Design review of the part shown in the three views and the two pictorial views. Dimensions are in mm from the part's minimum x, y and z. Give positions to 0.01 mm unless a question says otherwise; leave off trailing zeros. Loops run counter-clockwise (first coordinate to the right, second up) from the corner with the lowest first, then second, coordinate; pieces in that order, holes last. Notation, with made-up numbers: (-29.5, -16) -> (24.5, -16) arc R32 ccw to (24.5, 10) -> close; hole circle Ø2 at (85.25, 41.5). An arc over 180 degrees is marked (long way). Use CSV: the item, a comma, the result in double quotes. Start each with the question number.
Item 1: Wall thickness on line 1 along Y through (x, z) = (20.5, 67); line 2 along X through (y, z) = (14.25, 53); line 3 along X through (y, z) = (1, 57.5): over which ranges is each line inside the solid? List them lowest first. Write a range as from..to.
Item 2: The part is to be moulded in two halves that separate along Y. For the marked faces 1, 2, 3 and 4, say which applies: +Y half, -Y half, draft (parallel to the pull), parting line (faces both ways), or undercut.
Item 3: We need section D-D (y = 3). State the section outline as (x, z) points.
Item 4: We need section B-B (y = 9.5). State the section outline as (x, z) points, plus the area to 3 significant figures.
Item 5: We need section A-A (z = 6). State the section outline as (x, y) points.
Item 6: Clearance check with flat-ended pins moving along their axes: pin 1 (12 mm diameter, centred on y = 6, z = 50, fed in from +X); pin 2 (3 mm diameter, centred on x = 48, y = 8, fed in from +Z); pin 3 (8 mm diameter, centred on y = 10, z = 25, fed in from +X). State where each tip first meets the part, or that it passes through.
Item 7: We need section C-C (x = 67). State the section outline as (y, z) points.
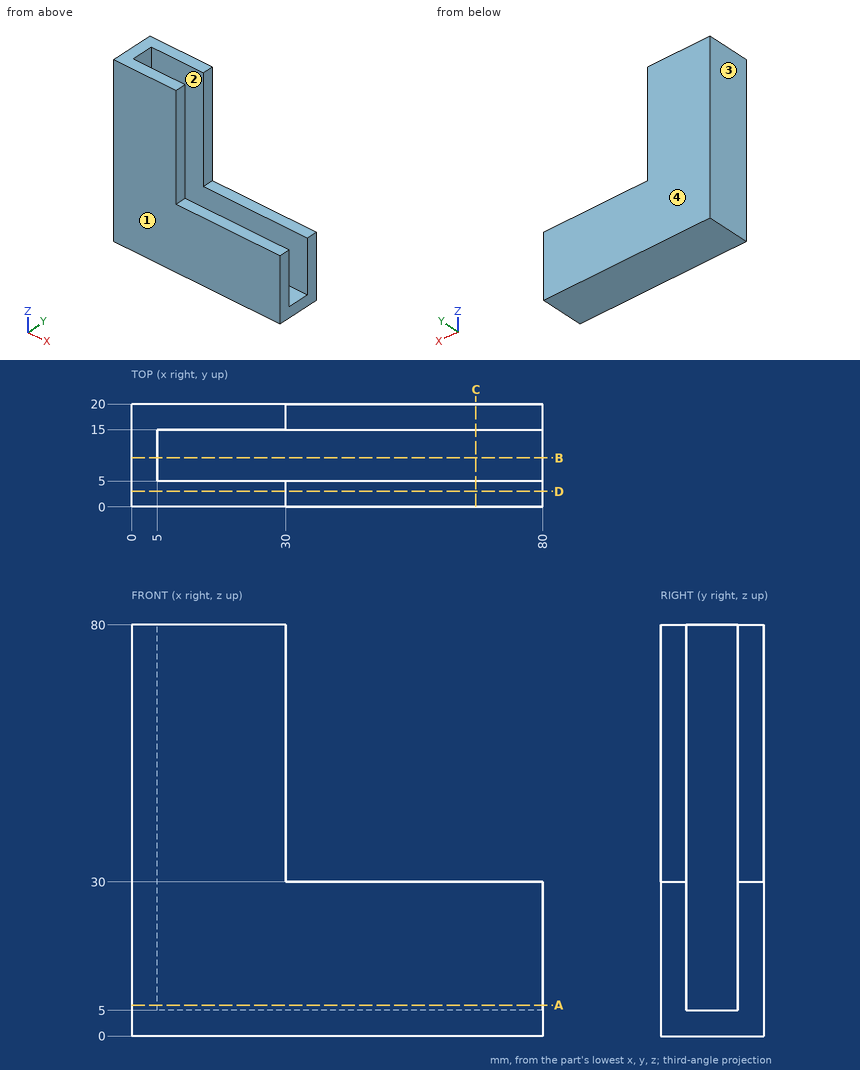
Results found:
1,line 1,"0..5, 15..20"
1,line 2,"0..5"
1,line 3,"0..30"
2,face 1,"-Y half"
2,face 2,"undercut"
2,face 3,"draft"
2,face 4,"+Y half"
3,outline,"(0, 0) -> (80, 0) -> (80, 30) -> (30, 30) -> (30, 80) -> (0, 80) -> close"
4,outline,"(0, 0) -> (80, 0) -> (80, 5) -> (5, 5) -> (5, 80) -> (0, 80) -> close"
4,area,"775 mm²"
5,outline,"(0, 0) -> (80, 0) -> (80, 5) -> (5, 5) -> (5, 15) -> (80, 15) -> (80, 20) -> (0, 20) -> close"
6,pin 1,"x = 30"
6,pin 2,"z = 5"
6,pin 3,"x = 5"
7,outline,"(0, 0) -> (20, 0) -> (20, 30) -> (15, 30) -> (15, 5) -> (5, 5) -> (5, 30) -> (0, 30) -> close"
